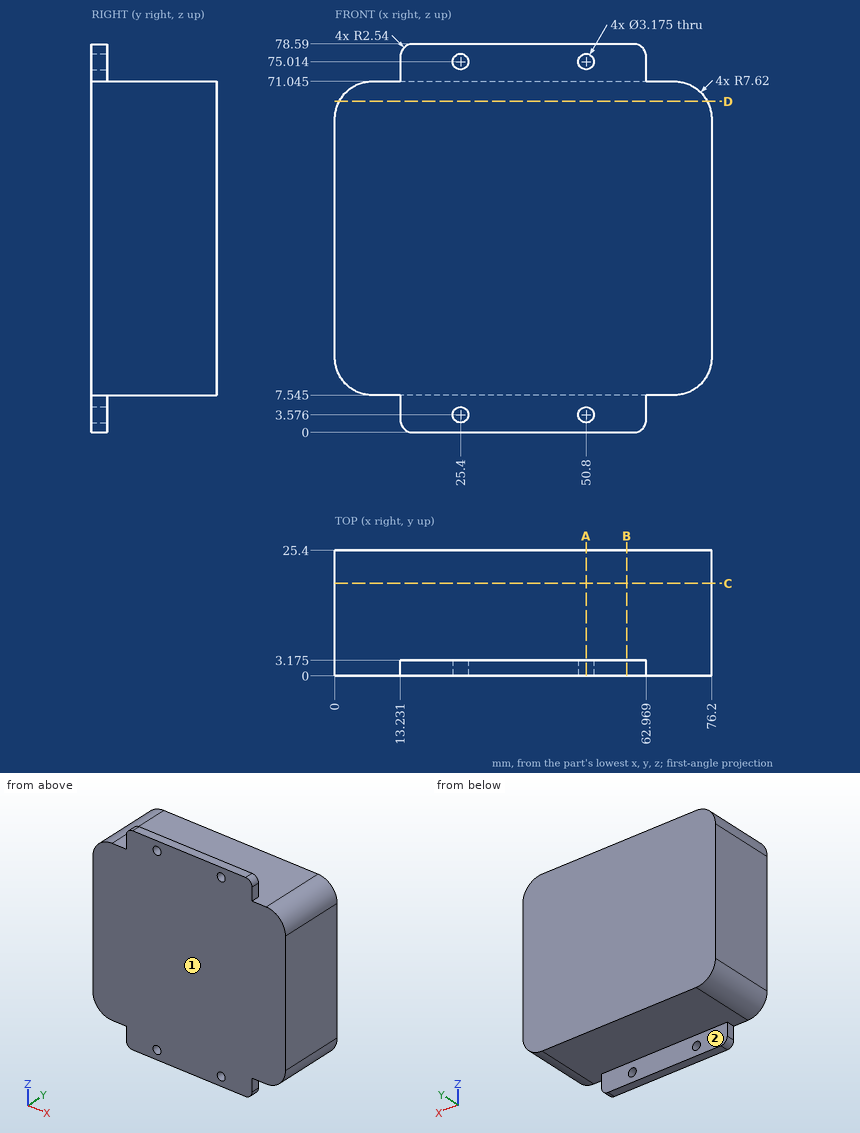
Check sheet for the drawn part. Datum: minimum x, y, z corner. Units: mm. A direction names the side the tool comes from. Give positions to 0.01 mm unless a question says otherwise; leave off trailing zeros. Loops run counter-clockwise (first coordinate to the right, second up) from the corner with the lowest first, then second, coordinate; pieces in that order, holes last. Notation, with made-up numbers: M -13.5,1 L 44.5,1 A15 ccw 44.5,25 Z; hole C 64,81 d3. An arc over 180 degrees is marked long. Return JSON: item names as keys, results as strings.
1) Section check C-C, the plane y = 18.75. Enter the section's corners in (x, z) (1 decimal), and give its area (3 significant figures).
Findings:
{"outline": "M 0,15.2 A7.6 ccw 7.6,7.5 L 68.6,7.5 A7.6 ccw 76.2,15.2 L 76.2,63.4 A7.6 ccw 68.6,71 L 7.6,71 A7.6 ccw 0,63.4 Z", "area": "4,790 mm2"}
2) Material ranges on L1, parallel to Z at x = 15, y = 6.75 (1 decimal); L2, parallel to Y at x = 45, z = 3 (1 decimal); L3, parallel to X at y = 21.75, z = 11.5, recorded low to high. Write a range as [from, to].
Findings:
{"L1": "z = [7.5, 71]", "L2": "y = [0, 3.2]", "L3": "x = [0.94, 75.26]"}
3) Section check D-D, the plane z = 67. Enter the section's corners in (x, y).
Findings:
{"outline": "M 0.89,0 L 75.31,0 L 75.31,25.4 L 0.89,25.4 Z"}
4) Gauge pin test, flat ends, axial feed: P1, Ø2.5, axis at y = 1.5, z = 4, coming from the -X side; P2, Ø12, axis at x = 15, y = 16.5, coming from the +Z side (1 decimal); P3, Ø10, axis at x = 38.5, y = 17, coming from the -Z side (1 decimal). Record the tip position at first contact, or that the pin passes through.
Findings:
{"P1": "stops at x = 13.23", "P2": "stops at z = 71", "P3": "stops at z = 7.5"}
5) Tool access check on the marked faces 1 and 2. Record the directions out of +Z, -Z, +X, -X, +Y, -Y that give a thin tool (end or side, any length) a straight path to the whole face; none if there is none.
Findings:
{"face 1": "+Z, -Z, +X, -X, -Y", "face 2": "-Z, +X, -X, +Y"}
6) Section check A-A, the plane x = 50.8. Enter the section's corners in (y, z) (1 decimal).
Findings:
{"outline": "M 0,0 L 3.2,0 L 3.2,2 L 0,2 Z; M 0,5.2 L 3.2,5.2 L 3.2,7.5 L 25.4,7.5 L 25.4,71 L 3.2,71 L 3.2,73.4 L 0,73.4 Z; M 0,76.6 L 3.2,76.6 L 3.2,78.6 L 0,78.6 Z"}
7) Section check B-B, the plane x = 59. Enter the section's corners in (y, z) (1 decimal).
Findings:
{"outline": "M 0,0 L 3.2,0 L 3.2,7.5 L 25.4,7.5 L 25.4,71 L 3.2,71 L 3.2,78.6 L 0,78.6 Z"}
